Geometry check sheet. Reference: the model listing, model coordinates, mm. Face numbers are marked on the shaded views. Give positions to 0.01 mm unless a question says otherwise; leave off trailing zeros. Write each loop counter-clockwise with the first axis right and the second up, starting at its lowest first coordinate (ties: lowest second). Pieces come first, ordered by that corner, then holes. Notation, with made-up numbers: (33, 16.5) -> (54, 16.5) arc R16 cw to (54, 44.5) -> close; hole circle Ø3 at (66.5, 79.5). An arc over 180 degrees is marked (long way). One line per item, written item: value.
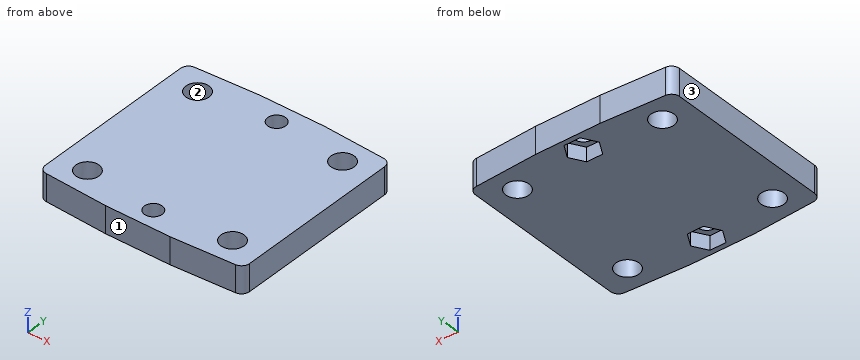
from build123d import *

# Parameters (mm, degrees)
SKETCH_R        = 4.3
PAD_DEPTH       = 10
SKETCH001_R     = 3.3
POCKET_DEPTH    = 10.001
POCKET001_DEPTH = 5.2
FILLET_R        = 3


with BuildPart() as part:
    # Sketch → Pad (new body)
    with BuildSketch(Plane.XY):
        Polygon((76, 0), (76, 67), (50, 68.5), (26, 68.5), (0, 67), (0, 0), (26, -1.5), (50, -1.5), align=None)
        with Locations((11, 58.5)):
            Circle(SKETCH_R, mode=Mode.SUBTRACT)
        with Locations((65, 58.5)):
            Circle(SKETCH_R, mode=Mode.SUBTRACT)
        with Locations((65, 8.5)):
            Circle(SKETCH_R, mode=Mode.SUBTRACT)
        with Locations((11, 8.5)):
            Circle(SKETCH_R, mode=Mode.SUBTRACT)
    extrude(amount=PAD_DEPTH)

    # Sketch001 (on Face14 of Pad) → Pocket (cut, through all)
    with BuildSketch(Plane.XY.offset(10)):
        with Locations((38, 61.5)):
            Circle(SKETCH001_R)
        with Locations((38, 5.5)):
            Circle(SKETCH001_R)
    extrude(amount=-POCKET_DEPTH, mode=Mode.SUBTRACT)

    # Sketch002 (on Face4 of Pocket) → Pocket001 (cut)
    with BuildSketch(Plane(origin=(0, 0, 0), x_dir=(1, 0, 0), z_dir=(0, 0, -1))):
        Polygon((40.973354, -10.65), (43.946708, -5.5), (40.973354, -0.35), (35.026646, -0.35), (32.053292, -5.5), (35.026646, -10.65), align=None)
        Polygon((43.946708, -61.5), (40.973354, -56.35), (35.026646, -56.35), (32.053292, -61.5), (35.026646, -66.65), (40.973354, -66.65), align=None)
    extrude(amount=-POCKET001_DEPTH, mode=Mode.SUBTRACT)

    # Fillet
    fillet_edges = [part.edges().sort_by_distance(p)[0] for p in [
        (0, 67, 5),
        (0, 0, 5),
        (76, 0, 5),
        (76, 67, 5),
    ]]
    fillet(fillet_edges, radius=FILLET_R)


solid = part.part
1) Sectioned sample at A-A on x = 38. Record the cut outline in (y, z).
Verdict:
outline: (-1.5, 0) -> (0.35, 0) -> (0.35, 5.2) -> (2.2, 5.2) -> (2.2, 10) -> (-1.5, 10) -> close; (8.8, 5.2) -> (10.65, 5.2) -> (10.65, 0) -> (56.35, 0) -> (56.35, 5.2) -> (58.2, 5.2) -> (58.2, 10) -> (8.8, 10) -> close; (64.8, 5.2) -> (66.65, 5.2) -> (66.65, 0) -> (68.5, 0) -> (68.5, 10) -> (64.8, 10) -> close
2) Sectioned sample at B-B on z = 3. Record the cut outline in (x, y), plus the area to 3 significant figures.
Verdict:
outline: (0, 2.83) arc R3 ccw to (2.83, -0.16) -> (26, -1.5) -> (50, -1.5) -> (73.17, -0.16) arc R3 ccw to (76, 2.83) -> (76, 64.17) arc R3 ccw to (73.17, 67.16) -> (50, 68.5) -> (26, 68.5) -> (2.83, 67.16) arc R3 ccw to (0, 64.17) -> close; hole circle Ø8.6 at (11, 8.5); hole circle Ø8.6 at (11, 58.5); hole (32.05, 5.5) -> (35.03, 0.35) -> (40.97, 0.35) -> (43.95, 5.5) -> (40.97, 10.65) -> (35.03, 10.65) -> close; hole (32.05, 61.5) -> (35.03, 56.35) -> (40.97, 56.35) -> (43.95, 61.5) -> (40.97, 66.65) -> (35.03, 66.65) -> close; hole circle Ø8.6 at (65, 8.5); hole circle Ø8.6 at (65, 58.5)
area: 4,820 mm^2
3) Sectioned sample at D-D on x = 64. Record the cut outline in (y, z).
Verdict:
outline: (-0.69, 0) -> (4.32, 0) -> (4.32, 10) -> (-0.69, 10) -> close; (12.68, 0) -> (54.32, 0) -> (54.32, 10) -> (12.68, 10) -> close; (62.68, 0) -> (67.69, 0) -> (67.69, 10) -> (62.68, 10) -> close
4) Sectioned sample at C-C on z = 7. Record the cut outline in (x, y), plus the area to 3 significant figures.
Verdict:
outline: (0, 2.83) arc R3 ccw to (2.83, -0.16) -> (26, -1.5) -> (50, -1.5) -> (73.17, -0.16) arc R3 ccw to (76, 2.83) -> (76, 64.17) arc R3 ccw to (73.17, 67.16) -> (50, 68.5) -> (26, 68.5) -> (2.83, 67.16) arc R3 ccw to (0, 64.17) -> close; hole circle Ø8.6 at (11, 8.5); hole circle Ø8.6 at (11, 58.5); hole circle Ø6.6 at (38, 5.5); hole circle Ø6.6 at (38, 61.5); hole circle Ø8.6 at (65, 8.5); hole circle Ø8.6 at (65, 58.5)
area: 4,930 mm^2
5) Scan lines: probe 1 along Y at (x, z) = (38, 7.4); probe 2 along Y at (x, z) = (65, 3.5); probe 3 along X at (y, z) = (5, 3.75). Record each from-to range of solid material in increasing order.
Verdict:
probe 1: -1.5 to 2.2, 8.8 to 58.2, 64.8 to 68.5
probe 2: -0.63 to 4.2, 12.8 to 54.2, 62.8 to 67.63
probe 3: 0 to 8.5, 13.5 to 32.34, 43.66 to 62.5, 67.5 to 76
6) Mould release check, pull along Y, two halves, no side actions. Record for the marked faces 1, 2 and 3: released by +Y, released by -Y, zero draft, split by the parting line, or undercut.
Verdict:
face 1: released by -Y
face 2: undercut
face 3: zero draft
7) Depth check by flat-ended pin: pin 1 Ø4 at (x, z) = (19.5, 4.5) entering from +Y. Enter the tip coordinate at first touch or a pass-through.
Verdict:
pin 1: y = 68.24
